Answer from the drawing. Dimensions are ordinates in mm from the lowest x, y and z of the part. Give positions to 0.01 mm unless a question says otherwise; leave off trailing zeros. Write each loop counter-clockwise with the first axis right and the second up, starting at its lowest first coordinate (ties: lowest second). Pieces come first, ordered by that corner, then holes.
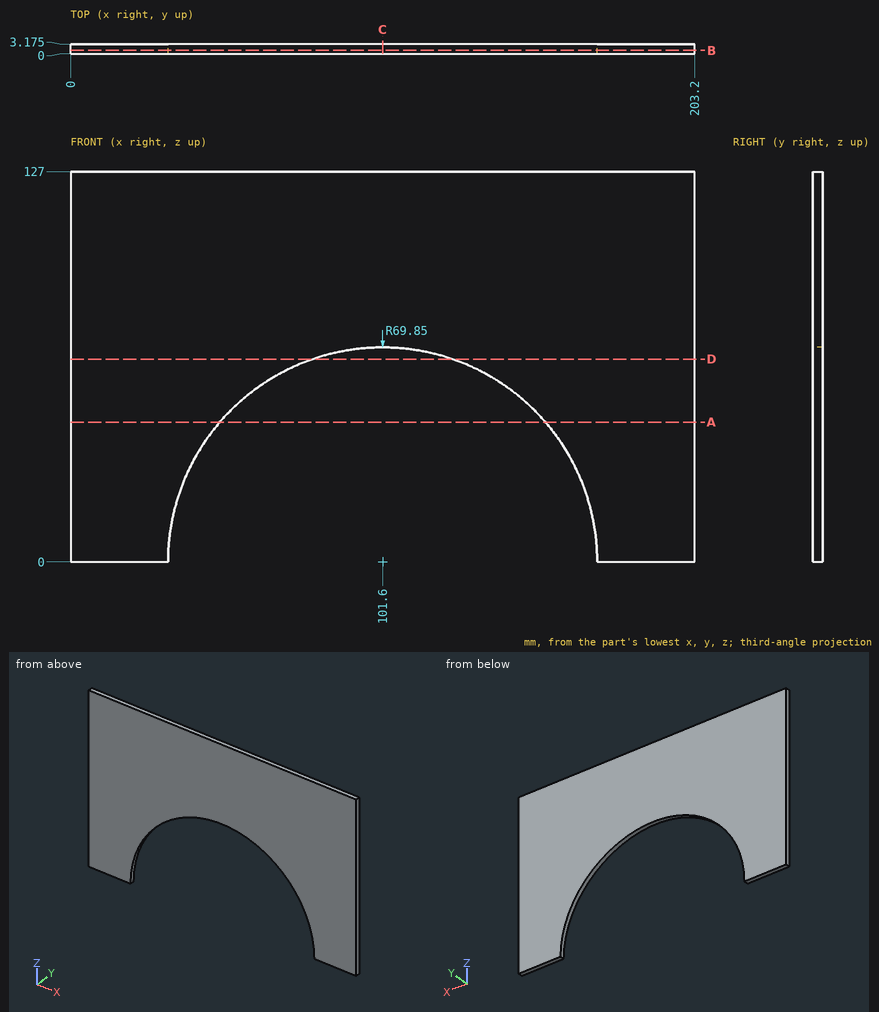
Item 1: Section C-C (x = 101.6) is taken. Write down the section's boundary in (y, z) (3 decimals), and give its area (3 significant figures).
Result set:
outline: (0, 69.85) - (3.175, 69.85) - (3.175, 127) - (0, 127) - close
area: 181 mm2
Item 2: Section B-B (y = 1.1) is taken. Write down the section's boundary in (x, z).
Result set:
outline: (0, 0) - (31.75, 0) arc R69.85 cw to (171.45, 0) - (203.2, 0) - (203.2, 127) - (0, 127) - close
Item 3: Section D-D (z = 66) is taken. Write down the section's boundary in (x, y) (3 decimals).
Result set:
outline: (0, 0) - (78.73, 0) - (78.73, 3.175) - (0, 3.175) - close; (124.47, 0) - (203.2, 0) - (203.2, 3.175) - (124.47, 3.175) - close
Item 4: Find the intervals of material crossed by line 1 along X through (y, z) = (2.4, 49.5); line 2 along X through (y, z) = (1.2, 8); line 3 along Z through (x, y) = (159, 1.35), in increasing order.
Result set:
line 1: x = 0 to 52.32, 150.88 to 203.2
line 2: x = 0 to 32.21, 170.99 to 203.2
line 3: z = 39.8 to 127
Item 5: Section A-A (z = 45.5) is taken. Write down the section's boundary in (x, y) (3 decimals).
Result set:
outline: (0, 0) - (48.602, 0) - (48.602, 3.175) - (0, 3.175) - close; (154.598, 0) - (203.2, 0) - (203.2, 3.175) - (154.598, 3.175) - close
